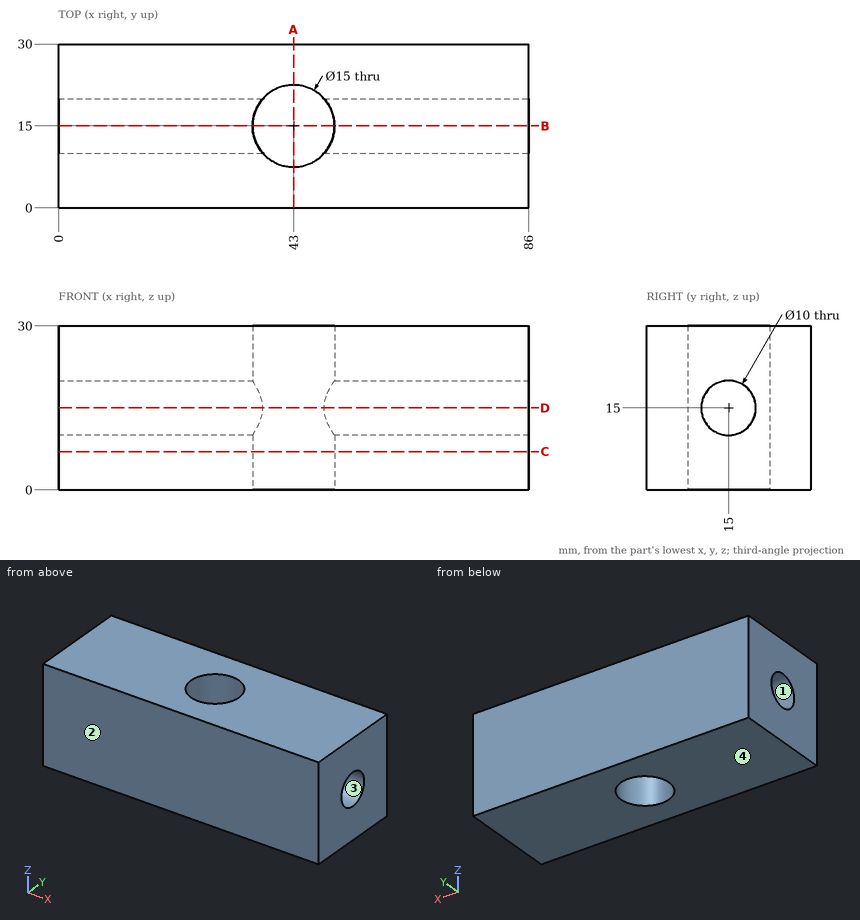
Input: dimensioned drawing with shaded views. Units: mm. Origin: part minimum x, y, z. Give positions to 0.01 mm unless a question says otherwise; leave off trailing zeros. Loops run counter-clockwise (first coordinate to the right, second up) from the corner with the lowest first, then second, coordinate; pieces in that order, holes last. Notation, with made-up numbers: (79.25, -2.75) -> (125.25, -2.75) arc R16 ccw to (125.25, 21.25) -> close; hole circle Ø8 at (45.5, 17.5). An arc over 180 degrees is marked (long way). Return JSON: item names as keys, results as strings.
Item 1: Section B-B, the plane y = 15. Output: boundary loops of the cut face in (x, z).
Filled in:
{"outline": "(0, 0) -> (35.5, 0) -> (35.5, 10) -> (0, 10) -> close; (0, 20) -> (35.5, 20) -> (35.5, 30) -> (0, 30) -> close; (50.5, 0) -> (86, 0) -> (86, 10) -> (50.5, 10) -> close; (50.5, 20) -> (86, 20) -> (86, 30) -> (50.5, 30) -> close"}
Item 2: Section D-D, the plane z = 15. Output: boundary loops of the cut face in (x, y), plus the area to 3 significant figures.
Filled in:
{"outline": "(0, 0) -> (86, 0) -> (86, 10) -> (48.59, 10) arc R7.5 cw to (37.41, 10) -> (0, 10) -> close; (0, 20) -> (37.41, 20) arc R7.5 cw to (48.59, 20) -> (86, 20) -> (86, 30) -> (0, 30) -> close", "area": "1,680 mm^2"}
Item 3: Line query: line 1 (X direction, y = 15, z = 8.5); line 2 (Y direction, x = 17, z = 15); line 3 (Y direction, x = 43, z = 8). Output: solid intervals per line, ascending.
Filled in:
{"line 1": "0 to 35.5, 50.5 to 86", "line 2": "0 to 10, 20 to 30", "line 3": "0 to 7.5, 22.5 to 30"}
Item 4: Section C-C, the plane z = 7. Output: boundary loops of the cut face in (x, y), plus the area to 3 significant figures.
Filled in:
{"outline": "(0, 0) -> (86, 0) -> (86, 30) -> (0, 30) -> close; hole circle Ø15 at (43, 15)", "area": "2,400 mm^2"}
Item 5: Mould query, pull axis Z, two halves, no side actions, for the marked faces 1, 2, 3 and 4. Classes: released by +Z, released by -Z, zero draft, split by the parting line, or undercut.
Filled in:
{"face 1": "undercut", "face 2": "zero draft", "face 3": "undercut", "face 4": "released by -Z"}
Item 6: Pin query (flat end, axial travel): P1, Ø2, axis at x = 36.5, z = 20, coming from the -Y side. Return the tip coordinate at first contact, or that it passes through.
Filled in:
{"P1": "y = 0"}
Item 7: Section A-A, the plane x = 43. Output: boundary loops of the cut face in (y, z).
Filled in:
{"outline": "(0, 0) -> (7.5, 0) -> (7.5, 30) -> (0, 30) -> close; (22.5, 0) -> (30, 0) -> (30, 30) -> (22.5, 30) -> close"}
